Answer from the drawing. Dimensions are ordinates in mm from the lowest x, y and z of the part. A direction names the side the tool comes from. Coordinates: 2 decimals unless noted, no trailing zeros. Write each loop counter-clockwise with the first axis right and the second up, starting at its lowest first coordinate (ties: lowest second). Pieces come first, ordered by that corner, then holes.
1) The part is cut by section B-B (x = 13). Give the number of separate pieces and of enclosed holes in the cut face.
2) Each of these flat-tipped pins is pushed along its axis until it touches: pin 1 Ø5 at (x, y) = (12.573, 12.573) entering from +Z; pin 2 Ø4 at (x, y) = (2.413, 12.573) entering from -Z; pin 3 Ø4 at (x, y) = (22.733, 12.573) entering from +Z; pin 4 Ø2 at (y, z) = (17, 1) entering from -X. Where does it stop, or does it pass through?
3) The part is cut by section C-C (x = 1.5). Determine the outline of the cut face in (y, z) (1 decimal).
4) Find the intervals of material crossed by line 1 (X direction, y = 11.75, z = 2.5) (1 decimal); line 2 (X direction, y = 13.75, z = 1.25) (1 decimal); line 3 (Y direction, x = 22.25, z = 1.6) (1 decimal), in increasing order.
5) Determine the mould class of the marked faces 3, 4 and 5 for opening direction Y: +Y half, -Y half, draft (parallel to the pull), parting line (faces both ways), or undercut.
6) The part is cut by section A-A (y = 22). Determine the outline of the cut face in (x, z) (1 decimal), then the cut area to 3 significant figures.
7) The part is cut by section D-D (y = 5.25). Determine the outline of the cut face in (x, z) (1 decimal).
8) Which of the six approach directions +Z, -Z, +X, -X, +Y, -Y give full straight-line access (tool end or side, diameter ignored) to the marked faces 1 and 2?
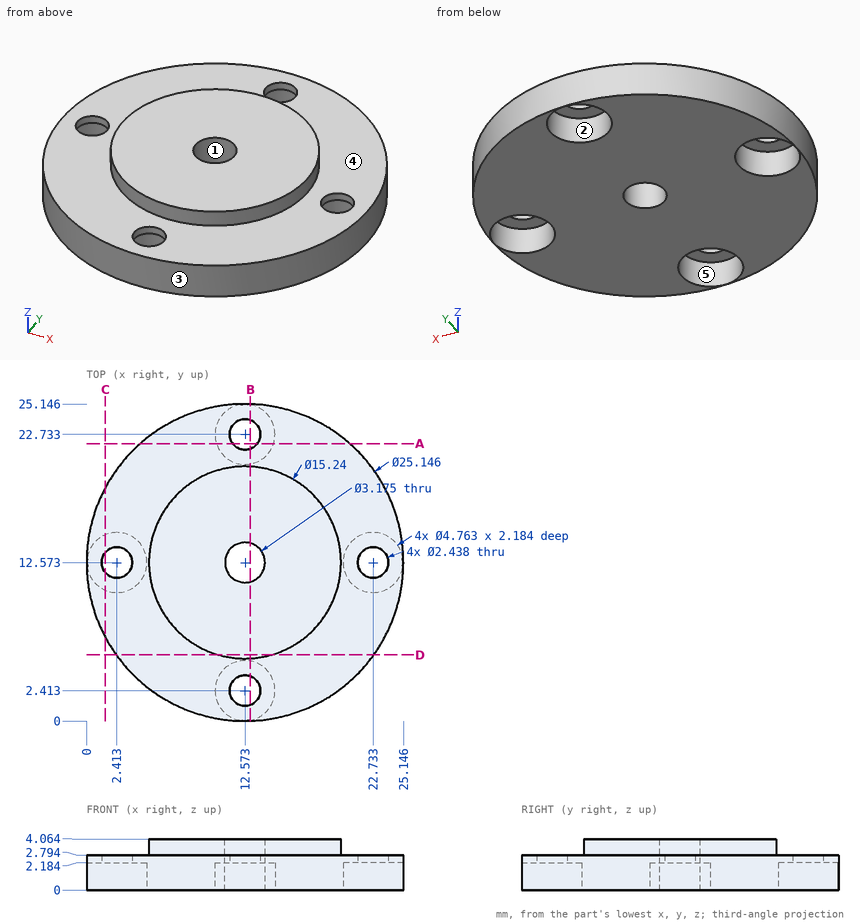
Reported:
1. separate pieces: 4
1. enclosed holes: 0
2. pin 1: stops at z = 4.06
2. pin 2: stops at z = 2.18
2. pin 3: stops at z = 2.79
2. pin 4: stops at x = 0.48
3. outline: (6.6, 0) - (10.4, 0) - (10.4, 2.2) - (11.8, 2.2) - (11.8, 2.8) - (6.6, 2.8) - close; (13.4, 2.2) - (14.8, 2.2) - (14.8, 0) - (18.5, 0) - (18.5, 2.8) - (13.4, 2.8) - close
4. line 1: x = 0 to 1.5, 3.3 to 11.2, 13.9 to 21.8, 23.6 to 25.1
4. line 2: x = 0.1 to 0.3, 4.5 to 11.5, 13.6 to 20.7, 24.8 to 25.1
4. line 3: y = 4.5 to 10.2, 14.9 to 20.6
5. face 3: parting line
5. face 4: draft
5. face 5: undercut
6. outline: (4.3, 0) - (10.3, 0) - (10.3, 2.2) - (11.6, 2.2) - (11.6, 2.8) - (4.3, 2.8) - close; (13.5, 2.2) - (14.8, 2.2) - (14.8, 0) - (20.9, 0) - (20.9, 2.8) - (13.5, 2.8) - close
6. area: 35.4 mm2
7. outline: (2.4, 0) - (22.8, 0) - (22.8, 2.8) - (14.7, 2.8) - (14.7, 4.1) - (10.5, 4.1) - (10.5, 2.8) - (2.4, 2.8) - close
8. face 1: +Z, -Z
8. face 2: -Z
